```python
from build123d import *

# Parameters (mm, degrees)
BOSS_EXTRU_1_DEPTH           = 3
ENL_V_MAT_EXTRU_1_DEPTH      = 117.633838487
ENL_V_MAT_EXTRU_1_DEPTH_BACK = 3
ENL_V_MAT_EXTRU_2_DEPTH      = 3
ESQUISSE4_W                  = 50
ESQUISSE4_H                  = 5
ENL_V_MAT_EXTRU_3_DEPTH      = 3


with BuildPart() as part:
    # Esquisse1 → Boss.-Extru.1 (new body)
    with BuildSketch(Plane.XY):
        Polygon((-78.272102247, -71.975308642), (31.727897753, 28.024691358), (91.727897753, 28.024691358), (91.727897753, -71.975308642), align=None)
    extrude(amount=BOSS_EXTRU_1_DEPTH)

    # Esquisse2 → Enlèv. mat.-Extru.1 (cut, two sides: drawn at the far end of the back side and taken through both)
    with BuildSketch(Plane.XY.offset(3).offset(-ENL_V_MAT_EXTRU_1_DEPTH_BACK)):
        Polygon((348.843028944, 207.929257012), (49.002086188, 28.024691358), (44.002086188, 25.024691358), (64.002086188, 25.024691358), (59.002086188, 28.024691358), (-240.838856568, 207.929257012), (-240.838856568, -491.413988315), (348.843028944, -491.413988315), align=None)
    extrude(amount=ENL_V_MAT_EXTRU_1_DEPTH + ENL_V_MAT_EXTRU_1_DEPTH_BACK, mode=Mode.SUBTRACT)

    # Esquisse3 → Enlèv. mat.-Extru.2 (cut)
    with BuildSketch(Plane.XY.offset(3)):
        Polygon((91.727897753, 8.024691358), (88.727897753, 13.024691358), (88.727897753, -6.975308642), (91.727897753, -1.975308642), align=None)
        Polygon((91.727897753, -41.975308642), (88.727897753, -36.975308642), (88.727897753, -56.975308642), (91.727897753, -51.975308642), align=None)
    extrude(amount=-ENL_V_MAT_EXTRU_2_DEPTH, mode=Mode.SUBTRACT)

    # Esquisse4 → Enlèv. mat.-Extru.3 (cut)
    with BuildSketch(Plane.XY.offset(3)):
        with Locations((7.568828052, -64.475308642)):
            Rectangle(ESQUISSE4_W, ESQUISSE4_H)
    extrude(amount=-ENL_V_MAT_EXTRU_3_DEPTH, mode=Mode.SUBTRACT)


solid = part.part
```
Could you check a few things on this model? Use its own coordinates, in mm. A direction names the side the tool comes from. Round coordinates to 2 decimals unless told otherwise and drop trailing zeros. Loops run counter-clockwise (first coordinate to the right, second up) from the corner with the lowest first, then second, coordinate; pieces in that order, holes last. Notation, with made-up numbers: M -2,67.5 L 51,67.5 A27 cw 51,83.5 Z; hole C 46.25,66.5 d2. An arc over 180 degrees is marked long. Answer as CSV lines item,"result".
1) We'd pull the mould along Y, two halves only. Please class faces 3 (the flat face through (91.728, 18, 1)), 4 (the flat face through (54, 25.025, 1)), 5 (the flat face through (75, 28.025, 1)): released by +Y, released by -Y, zero draft, split by the parting line, or undercut.
From the geometry:
face 3,"zero draft"
face 4,"undercut"
face 5,"released by +Y"
2) Imagine slicing it at B-B on x = -2. List the corners of the cut face in (y, z) for me, and give its area (3 significant figures).
From the geometry:
outline,"M -71.98,0 L -66.98,0 L -66.98,3 L -71.98,3 Z; M -61.98,0 L -2.64,0 L -2.64,3 L -61.98,3 Z"
area,"193 mm^2"
3) If I drill on probe 1 along X at (y, z) = (-55.5, 2.85); probe 2 along X at (y, z) = (-39, 1.45); probe 3 along Y at (x, z) = (-10, 1.9), over which ranges is the centre line in solid material (lowest first)?
From the geometry:
probe 1,"-60.15 to 88.73, 89.61 to 91.73"
probe 2,"-42 to 88.73, 89.94 to 91.73"
probe 3,"-71.98 to -66.98, -61.98 to -9.91"
4) For pin 1 Ø0.9 at (x, z) = (16, 1) entering from +Y; pin 2 Ø1.5 at (y, z) = (-49.5, 1.5) entering from +X; pin 3 Ø1 at (x, z) = (-2.5, 0.5) entering from +Y, each with a flat end and sliding along its axis, tell me the tip position at first contact or that it passes through.
From the geometry:
pin 1,"y = 14.14"
pin 2,"x = 88.73"
pin 3,"y = -2.64"
5) Which directions (+Z, -Z, +X, -X, +Y, -Y) give clear straight access to the entire face, cutting with the end or side of a thin tool? Please do faces 1 (the flat face through (91.728, -62, 1)), 2 (the flat face through (7, -66.975, 2)).
From the geometry:
face 1,"+Z, -Z, +X, +Y, -Y"
face 2,"+Z, -Z"
6) Imagine slicing it at C-C on y = -12.5. List the corners of the cut face in (x, z) for me.
From the geometry:
outline,"M -12.85,0 L 91.73,0 L 91.73,3 L -12.85,3 Z"
7) Imagine slicing it at D-D on x = 15. List the corners of the cut face in (y, z) for me.
From the geometry:
outline,"M -71.98,0 L -66.98,0 L -66.98,3 L -71.98,3 Z; M -61.98,0 L 12.82,0 L 12.82,3 L -61.98,3 Z"
8) Imagine slicing it at A-A on z = 1.7. List the corners of the cut face in (x, y) for me.
From the geometry:
outline,"M -78.27,-71.98 L 91.73,-71.98 L 91.73,-51.98 L 88.73,-56.98 L 88.73,-36.98 L 91.73,-41.98 L 91.73,-1.98 L 88.73,-6.98 L 88.73,13.02 L 91.73,8.02 L 91.73,28.02 L 59,28.02 L 64,25.02 L 44,25.02 L 49,28.02 L 31.73,28.02 Z; hole M -17.43,-66.98 L 32.57,-66.98 L 32.57,-61.98 L -17.43,-61.98 Z"
